The listing builds one solid part. Answer for the finished solid, in the listing's coordinates (mm). A direction names the side the tool comes from. Give positions to 0.01 mm unless a question says otherwise; leave off trailing zeros. Order: outer loops, then holes, each group sorted by start corner. A loop starts at its lowest first (then second) coordinate and runs counter-clockwise, first axis right, second up.
```python
from build123d import *

# Parameters (mm, degrees)
SKETCH1_W                   = 25
SKETCH1_H                   = 250
M8_TAPPED_HOLE1_D           = 6.8
M8_TAPPED_HOLE1_DEPTH       = 16.75
M8_TAPPED_HOLE1_CSINK_D     = 8.05
M8_TAPPED_HOLE1_CSINK_ANGLE = 90
M8_TAPPED_HOLE1_TIP         = 2.042926105
FILLET1_R                   = 2.5


with BuildPart() as part:
    # Sketch1 → Revolve1 (revolve)
    with BuildSketch(Plane.XY, mode=Mode.PRIVATE) as revolve1_sk:
        with Locations((12.5, 125)):
            Rectangle(SKETCH1_W, SKETCH1_H)
    revolve(revolve1_sk.sketch.rotate(Axis((0, 0, 0), (0, 1, 0)), 90), axis=Axis((0, 0, 0), (0, 1, 0)))

    # M8 Tapped Hole1
    with Locations(Plane.ZX.offset(250)):
        with Locations((0, 0)):
            CounterSinkHole(M8_TAPPED_HOLE1_D / 2, M8_TAPPED_HOLE1_CSINK_D / 2, depth=M8_TAPPED_HOLE1_DEPTH, counter_sink_angle=M8_TAPPED_HOLE1_CSINK_ANGLE)
            with Locations((0, 0, -(M8_TAPPED_HOLE1_DEPTH + M8_TAPPED_HOLE1_TIP / 2))):  # 118° drill point
                Cone(0, M8_TAPPED_HOLE1_D / 2, M8_TAPPED_HOLE1_TIP, mode=Mode.SUBTRACT)

    # Fillet1
    fillet1_edges = [part.edges().sort_by_distance(p)[0] for p in [
        (0, 250, 25),
    ]]
    fillet(fillet1_edges, radius=FILLET1_R)


solid = part.part
```
1) For a pull along Z with two mould halves and no side action, classify faces 3 (the flat face through (5, 250, 0)), 4 (the conical face through (-0.576, 231.562, -0.128)), 5 (the cylindrical face through (-7.509, 125.482, -23.846)) as +Z half, -Z half, draft (parallel to the pull), parting line (faces both ways), or undercut.
Geometry says:
face 3: draft
face 4: undercut
face 5: parting line
2) A tool of negligible diameter and unlimited length cuts with its end or side. For faces 1 (the cylindrical face through (-3.32, 241.2, 0.74)), 2 (the flat face through (0, 0, 0)), from which of +Z, -Z, +X, -X, +Y, -Y can it reach the whole face along a straight path? Write none if from no direction.
Geometry says:
face 1: +Y
face 2: +Z, -Z, +X, -X, -Y
3) Straight lines are drawn through the part: probe 1 along X at (y, z) = (240.5, 0); probe 2 along Y at (x, z) = (3, -1.5); probe 3 along X at (y, z) = (59, -1). For each, find the intervals that lie inside material, in ascending order.
Geometry says:
probe 1: x = -25 to -3.4, 3.4 to 25
probe 2: y = 0 to 233.22
probe 3: x = -24.98 to 24.98
4) Given P1, Ø6, axis at y = 139, z = 2, coming from the +X side; P2, Ø1.5, axis at x = -10.5, y = 60, coming from the +Z side; P3, Ø8, axis at x = 0, z = 0, coming from the -Y side; P4, Ø12, axis at y = 75, z = 8, coming from the +X side, each flat-ended and moving along its own axis, determine where each tip first touches the part or whether it passes through.
Geometry says:
P1: stops at x = 25
P2: stops at z = 23.02
P3: stops at y = 0
P4: stops at x = 24.92
5) Find section A-A (y = 112.5). Write down the section's boundary in (x, z).
Geometry says:
outline: circle Ø50 at (0, 0)
